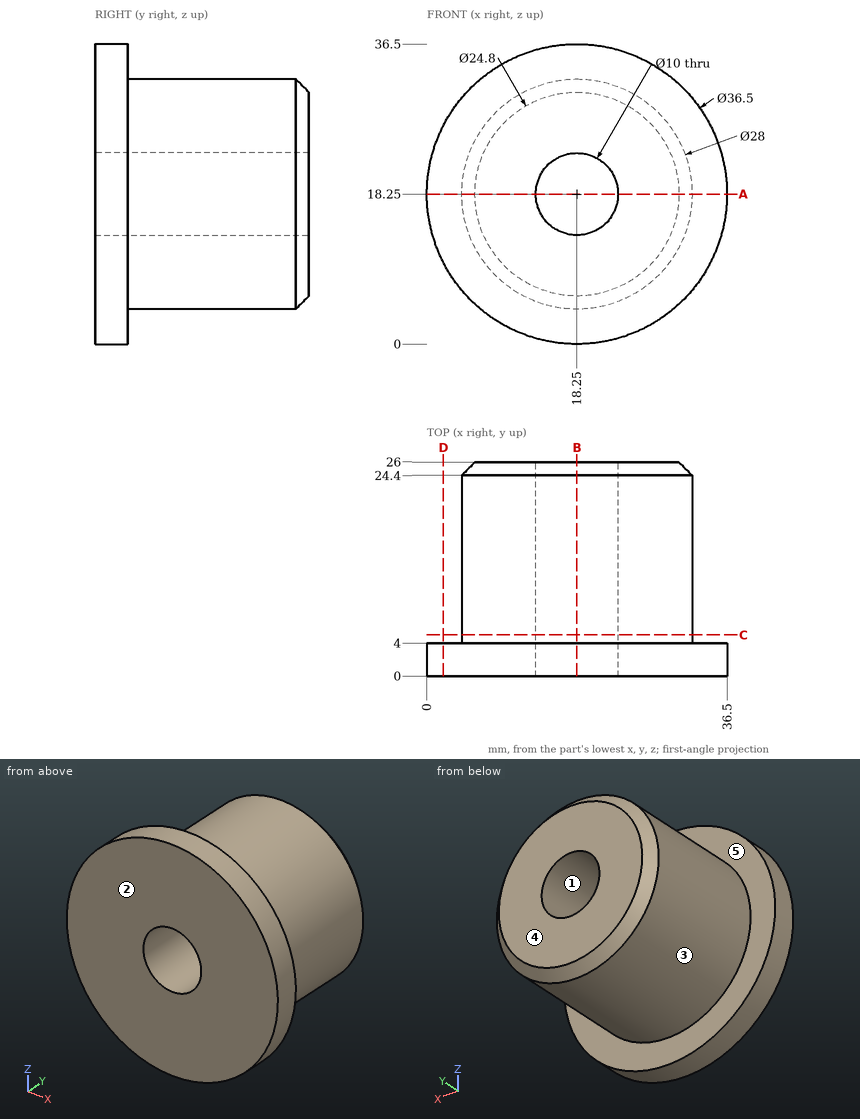
Geometry check sheet. Reference: drawing and pictorial views, mm from the part's lowest x, y, z. A direction names the side the tool comes from. Coordinates: 2 decimals unless noted, no trailing zeros. Loops run counter-clockwise (first coordinate to the right, second up) from the corner with the lowest first, then second, coordinate; pieces in that order, holes last. Notation, with made-up numbers: M 27,-40 L 76,-40 A7 cw 76,-28 Z; hole C 23.5,53 d7. An arc over 180 degrees is marked long. One line per item, written item: value.
1. Set-up check for the marked faces 4 and 5: record each of +Z, -Z, +X, -X, +Y, -Y from which the full face is reachable in a straight line by a thin tool's end or side.
Answers follow:
face 4: +Z, -Z, +X, -X, +Y
face 5: +Y
2. Section check D-D on x = 2. Record the cut outline in (y, z), plus the area to 3 significant figures.
Answers follow:
outline: M 0,9.94 L 4,9.94 L 4,26.56 L 0,26.56 Z
area: 66.5 mm^2
3. Section check A-A on z = 18.25. Record the cut outline in (x, y), plus the area to 3 significant figures.
Answers follow:
outline: M 0,0 L 13.25,0 L 13.25,26 L 5.85,26 L 4.25,24.4 L 4.25,4 L 0,4 Z; M 23.25,0 L 36.5,0 L 36.5,4 L 32.25,4 L 32.25,24.4 L 30.65,26 L 23.25,26 Z
area: 499 mm^2
4. Gauge pin test, flat ends, axial feed: P1, Ø2, axis at x = 26.5, y = 20.5, coming from the +Z side; P2, Ø10, axis at y = 12.5, z = 20, coming from the +X side; P3, Ø8, axis at x = 21.5, y = 11.5, coming from the -Z side. Record the tip position at first contact, or that the pin passes through.
Answers follow:
P1: z = 30.23
P2: x = 32.25
P3: z = 4.25
5. Section check C-C on y = 5. Record the cut outline in (x, z), plus the area to 3 significant figures.
Answers follow:
outline: C 18.25,18.25 d28; hole C 18.25,18.25 d10
area: 537 mm^2
6. Mould release check, pull along X, two halves, no side actions. Record for the marked faces 1, 2 and 3: pulls with the +X half, pulls with the -X half, needs draft (parallel to the pull), parting line crosses it, or undercut.
Answers follow:
face 1: undercut
face 2: needs draft
face 3: parting line crosses it
7. Section check B-B on x = 18.25. Record the cut outline in (y, z).
Answers follow:
outline: M 0,0 L 4,0 L 4,4.25 L 24.4,4.25 L 26,5.85 L 26,13.25 L 0,13.25 Z; M 0,23.25 L 26,23.25 L 26,30.65 L 24.4,32.25 L 4,32.25 L 4,36.5 L 0,36.5 Z
8. Material ranges on line 1 along X through (y, z) = (20.5, 18.25); line 2 along Y through (x, z) = (24, 33.5); line 3 along X through (y, z) = (19.5, 16), recorded low to high. Write a range as from..to.
Answers follow:
line 1: 4.25..13.25, 23.25..32.25
line 2: 0..4
line 3: 4.43..13.78, 22.72..32.07
